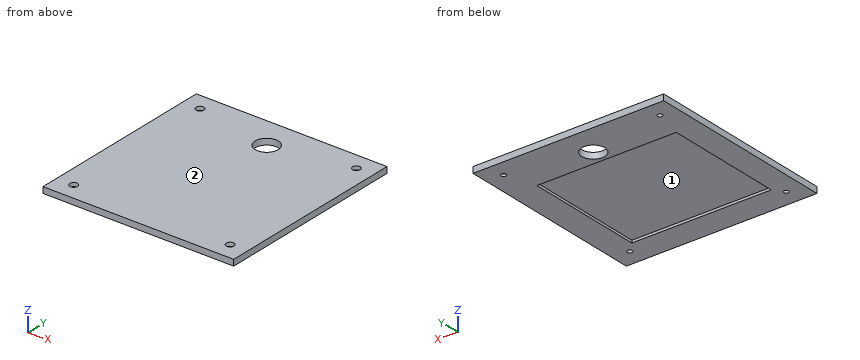
```python
from build123d import *

# Parameters (mm, degrees)
SKETCH_213_W        = 78
SKETCH_213_H        = 79
EXTRUDE_3_DEPTH     = 2.5
CUT_EXTRUDE_4_REACH = 59.522
SKETCH_10_R         = 1.00000254
SKETCH_10_R_2       = 4.7
CUT_EXTRUDE_START   = 1
SKETCH_12_R         = 1.6
CUT_EXTRUDE_6_DEPTH = 2.5
SKETCH_11_W         = 57.00006223
SKETCH_11_H         = 48.946928069
CUT_EXTRUDE_7_DEPTH = 1


with BuildPart() as part:
    # Sketch 213 → Extrude 3 (new body)
    with BuildSketch(Plane.XY):
        with Locations((1.76392246, -1.007858704)):
            Rectangle(SKETCH_213_W, SKETCH_213_H)
    extrude(amount=EXTRUDE_3_DEPTH)

    # Sketch 10 → Cut-Extrude 4 (cut, up to next)
    with BuildSketch(Plane.XY, mode=Mode.PRIVATE) as cut_extrude_4_sk1:
        with Locations(Location((-30.179759278, 31.492141296, 0), (0, 0, 180))):
            Circle(SKETCH_10_R)
    cut_extrude_4_tool1 = extrude(cut_extrude_4_sk1.sketch, amount=CUT_EXTRUDE_4_REACH, mode=Mode.PRIVATE) & part.part
    # Sketch 10 → Cut-Extrude 4 (cut, up to next)
    with BuildSketch(Plane.XY, mode=Mode.PRIVATE) as cut_extrude_4_sk2:
        with Locations(Location((33.76398723, 31.492283536, 0), (0, 0, 180))):
            Circle(SKETCH_10_R)
    cut_extrude_4_tool2 = extrude(cut_extrude_4_sk2.sketch, amount=CUT_EXTRUDE_4_REACH, mode=Mode.PRIVATE) & part.part
    # Sketch 10 → Cut-Extrude 4 (cut, up to next)
    with BuildSketch(Plane.XY, mode=Mode.PRIVATE) as cut_extrude_4_sk3:
        with Locations(Location((33.76398723, -33.507848544, 0), (0, 0, 180))):
            Circle(SKETCH_10_R)
    cut_extrude_4_tool3 = extrude(cut_extrude_4_sk3.sketch, amount=CUT_EXTRUDE_4_REACH, mode=Mode.PRIVATE) & part.part
    # Sketch 10 → Cut-Extrude 4 (cut, up to next)
    with BuildSketch(Plane.XY, mode=Mode.PRIVATE) as cut_extrude_4_sk4:
        with Locations(Location((-30.23614231, -33.507848544, 0), (0, 0, 180))):
            Circle(SKETCH_10_R)
    cut_extrude_4_tool4 = extrude(cut_extrude_4_sk4.sketch, amount=CUT_EXTRUDE_4_REACH, mode=Mode.PRIVATE) & part.part
    # Sketch 10 → Cut-Extrude 4 (cut, up to next)
    with BuildSketch(Plane.XY, mode=Mode.PRIVATE) as cut_extrude_4_sk5:
        with Locations(Location((1.764114511, 25.639082065, 0), (0, 0, 180))):
            Circle(SKETCH_10_R_2)
    cut_extrude_4_tool5 = extrude(cut_extrude_4_sk5.sketch, amount=CUT_EXTRUDE_4_REACH, mode=Mode.PRIVATE) & part.part
    add(cut_extrude_4_tool1.solids().sort_by_distance((-30.179759, 31.492141, 0))[0], mode=Mode.SUBTRACT)
    add(cut_extrude_4_tool2.solids().sort_by_distance((33.763987, 31.492284, 0))[0], mode=Mode.SUBTRACT)
    add(cut_extrude_4_tool3.solids().sort_by_distance((33.763987, -33.507849, 0))[0], mode=Mode.SUBTRACT)
    add(cut_extrude_4_tool4.solids().sort_by_distance((-30.236142, -33.507849, 0))[0], mode=Mode.SUBTRACT)
    add(cut_extrude_4_tool5.solids().sort_by_distance((1.764115, 25.639082, 0))[0], mode=Mode.SUBTRACT)

    # Sketch 12 → Cut-Extrude 6 (cut)
    with BuildSketch(Plane.XY.offset(CUT_EXTRUDE_START)):
        with Locations(Location((-30.179759278, 31.492141296, 0), (0, 0, 180))):
            Circle(SKETCH_12_R)
        with Locations(Location((33.76398723, 31.492283536, 0), (0, 0, 180))):
            Circle(SKETCH_12_R)
        with Locations(Location((-30.23614231, -33.507848544, 0), (0, 0, 180))):
            Circle(SKETCH_12_R)
        with Locations(Location((33.76398723, -33.507848544, 0), (0, 0, 180))):
            Circle(SKETCH_12_R)
    extrude(amount=CUT_EXTRUDE_6_DEPTH, mode=Mode.SUBTRACT)

    # Sketch 11 → Cut-Extrude 7 (cut)
    with BuildSketch(Plane(origin=(0, 0, 0), x_dir=(-1, 0, 0), z_dir=(0, 0, -1))):
        with Locations((-1.263953575, -5.03438197)):
            Rectangle(SKETCH_11_W, SKETCH_11_H)
    extrude(amount=-CUT_EXTRUDE_7_DEPTH, mode=Mode.SUBTRACT)


solid = part.part
```
Verification items for the finished model (mm, model axes). Face numbers are marked on the shaded views. A direction names the side the tool comes from. Coordinates: 2 decimals unless noted, no trailing zeros. Loops run counter-clockwise (first coordinate to the right, second up) from the corner with the lowest first, then second, coordinate; pieces in that order, holes last. Notation, with made-up numbers: (42.25, -11) - (75.25, -11) arc R32 cw to (75.25, 19) - close; hole circle Ø6 at (46.25, -3.75). An arc over 180 degrees is marked (long way). Answer as a JSON object with one key per item and string values.
(1) Cross-section at A-A, the plane x = -5. Record the boundary of the cut face in (y, z).
Response:
{"outline": "(-40.51, 0) - (-29.51, 0) - (-29.51, 1) - (19.44, 1) - (19.44, 0) - (38.49, 0) - (38.49, 2.5) - (-40.51, 2.5) - close"}
(2) Cross-section at B-B, the plane y = 10. Record the boundary of the cut face in (x, z).
Response:
{"outline": "(-37.24, 0) - (-27.24, 0) - (-27.24, 1) - (29.76, 1) - (29.76, 0) - (40.76, 0) - (40.76, 2.5) - (-37.24, 2.5) - close"}
(3) Access from +Z, -Z, +X, -X, +Y, -Y to the whole of each face (thin tool, end or side, straight path). Record for the marked faces 1 and 2.
Response:
{"face 1": "-Z", "face 2": "+Z, +X, -X, +Y, -Y"}
(4) Go/stop test with flat-tipped pins: pin 1 Ø2.5 at (x, y) = (-30.18, 31.49) entering from +Z; pin 2 Ø1 at (x, y) = (10.5, -11.5) entering from -Z. Record where each tip stops, or that it passes through.
Response:
{"pin 1": "stops at z = 1", "pin 2": "stops at z = 1"}
(5) Cross-section at D-D, the plane y = 23.5. Record the boundary of the cut face in (x, z), then the cut area to 3 significant figures.
Response:
{"outline": "(-37.24, 0) - (-2.42, 0) - (-2.42, 2.5) - (-37.24, 2.5) - close; (5.95, 0) - (40.76, 0) - (40.76, 2.5) - (5.95, 2.5) - close", "area": "174 mm²"}
(6) Scan lines: line 1 along X through (y, z) = (13, 0.55); line 2 along Y through (x, z) = (-25.5, 0.45); line 3 along Z through (x, y) = (-8, 10). Record each from-to range of solid material in increasing order.
Response:
{"line 1": "x = -37.24 to -27.24, 29.76 to 40.76", "line 2": "y = -40.51 to -29.51, 19.44 to 38.49", "line 3": "z = 1 to 2.5"}
(7) Cross-section at C-C, the plane z = 0.5. Record the boundary of the cut face in (x, y), then the cut area to 3 significant figures.
Response:
{"outline": "(-37.24, -40.51) - (40.76, -40.51) - (40.76, 38.49) - (-37.24, 38.49) - close; hole circle Ø2 at (-30.24, -33.51); hole circle Ø2 at (-30.18, 31.49); hole (-27.24, -29.51) - (29.76, -29.51) - (29.76, 19.44) - (-27.24, 19.44) - close; hole circle Ø9.4 at (1.76, 25.64); hole circle Ø2 at (33.76, -33.51); hole circle Ø2 at (33.76, 31.49)", "area": "3,290 mm²"}
